Build history of the part. All positions in model axes, mm. Face numbers are marked on the shaded views. A direction names the side the tool comes from. Give positions to 0.01 mm unless a question says otherwise; leave off trailing zeros. Loops run counter-clockwise (first coordinate to the right, second up) from the corner with the lowest first, then second, coordinate; pieces in that order, holes last.
1) Flat gauge pins, fed straight in: P1, Ø4, axis at x = -778, z = -243, coming from the -Y side; P2, Ø2.5, axis at x = 86.5, y = 228, coming from the +Z side. Where does each tip first touch, or does it go through?
2) Band-saw the part on C-C on z = 38.5. List the corners of the cut face in (x, y).
3) Wall check: line 1 (X direction, y = 161, z = -438); line 2 (Y direction, x = 46, z = -27.5); line 3 (Y direction, x = 5, z = 47). Give the ranges that are in metal, low to high.
4) 3-axis set-ups, long thin cutter, end or side, ignore diameter. For the marked faces 4, 5, 6 and 7: which of +Z, -Z, +X, -X, +Y, -Y reach the whole face in a straight line?
5) Band-saw the part on A-A on x = -13. List the corners of the cut face in (y, z), then the cut area to 4 significant figures.
6) Band-saw the part on D-D on y = 107. List the corners of the cut face in (x, z), then the cut area to 3 significant figures.
7) Band-saw the part on B-B on y = -146.5. List the corners of the cut face in (x, z).
8) Two-plate mould, pull along X, no slides. Class the marked faces 1, 2 and 3: +X half, -X half, draft (parallel to the pull), parting line (faces both ways), or undercut.
```python
from build123d import *

# Parameters (mm, degrees)
F0_W      = 1560
F0_H      = 450
F0_W_2    = 1440
F0_H_2    = 330
F1_DEPTH  = 90
F3_DEPTH  = 505
F4_W      = 1560
F4_H      = 5
F6_DEPTH  = 10
F5_W      = 1560
F5_H      = 5
F7_DEPTH  = 10
F9_DEPTH  = 10
F11_DEPTH = 10


with BuildPart() as f1:
    # F0 (on Top) → F1 (new body)
    with BuildSketch(Plane.XY):
        Rectangle(F0_W, F0_H)
        Rectangle(F0_W_2, F0_H_2, mode=Mode.SUBTRACT)
    extrude(amount=F1_DEPTH)

    # F2 (on face) → F3 (join)
    with BuildSketch(Plane(origin=(0, 0, 0), x_dir=(1, 0, 0), z_dir=(0, 0, -1))):
        Polygon((-780, 225), (-780, 125), (-775, 125), (-775, 220), (-680, 220), (-680, 225), align=None)
        Polygon((-775, -125), (-780, -125), (-780, -225), (-680, -225), (-680, -220), (-775, -220), align=None)
        Polygon((50, 225), (-50, 225), (-50, 175), (-45, 175), (-45, 220), (50, 220), align=None)
        Polygon((-50, -220), (-50, -225), (50, -225), (50, -175), (45, -175), (45, -220), align=None)
        Polygon((780, 225), (680, 225), (680, 220), (775, 220), (775, 125), (780, 125), align=None)
        Polygon((680, -220), (680, -225), (780, -225), (780, -125), (775, -125), (775, -220), align=None)
    extrude(amount=F3_DEPTH)

    # F4 (on face) → F6 (join)
    with BuildSketch(Plane.XZ.offset(225)):
        with Locations((0, 2.5)):
            Rectangle(F4_W, F4_H)
    extrude(amount=F6_DEPTH)

    # F5 (on face) → F7 (join)
    with BuildSketch(Plane(origin=(0, 225, 0), x_dir=(-1, 0, 0), z_dir=(0, 1, 0))):
        with Locations((0, 2.5)):
            Rectangle(F5_W, F5_H)
    extrude(amount=F7_DEPTH)

    # F8 (on face) → F9 (join)
    with BuildSketch(Plane.XY.offset(5)):
        Polygon((-780, -230), (-780, -235), (-775, -235), (775, -235), (780, -235), (780, -230), (780, -225), (775, -225), (775, -230), (-775, -230), (-775, -225), (-780, -225), align=None)
    extrude(amount=F9_DEPTH)

    # F10 (on face) → F11 (join)
    with BuildSketch(Plane.XY.offset(5)):
        Polygon((-780, 235), (-780, 225), (-775, 225), (-775, 230), (775, 230), (775, 225), (780, 225), (780, 230), (780, 235), (-775, 235), align=None)
    extrude(amount=F11_DEPTH)


solid = f1.part
```
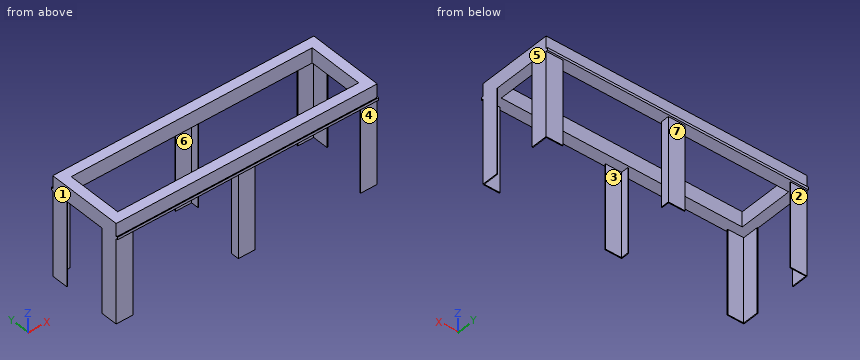
Findings below:
1. P1: stops at y = -225
1. P2: stops at z = 5
2. outline: (-780, -225) - (780, -225) - (780, 225) - (-780, 225) - close; hole (-720, -165) - (720, -165) - (720, 165) - (-720, 165) - close
3. line 1: x = -780 to -775, 775 to 780
3. line 2: y = -225 to -220, 175 to 225
3. line 3: y = -225 to -165, 165 to 225
4. face 4: -Z, +X, -X, -Y
4. face 5: +Z, -Z, +X, +Y, -Y
4. face 6: -Z
4. face 7: -Z, +X, -X, +Y
5. outline: (-235, 0) - (-225, 0) - (-225, -505) - (-220, -505) - (-220, 0) - (-165, 0) - (-165, 90) - (-225, 90) - (-225, 5) - (-230, 5) - (-230, 15) - (-235, 15) - close; (165, 0) - (220, 0) - (220, -505) - (225, -505) - (225, 0) - (235, 0) - (235, 15) - (230, 15) - (230, 5) - (225, 5) - (225, 90) - (165, 90) - close
5. area: 16,050 mm2
6. outline: (-780, 0) - (-720, 0) - (-720, 90) - (-780, 90) - close; (720, 0) - (780, 0) - (780, 90) - (720, 90) - close
6. area: 10,800 mm2
7. outline: (-780, -505) - (-775, -505) - (-775, 0) - (-720, 0) - (-720, 90) - (-780, 90) - close; (720, 0) - (775, 0) - (775, -505) - (780, -505) - (780, 90) - (720, 90) - close
8. face 1: -X half
8. face 2: draft
8. face 3: undercut
